```python
from build123d import *

# Parameters (mm, degrees)
BLANKSKE_W              = 85
BLANKSKE_H              = 12.5
BLANK_DEPTH             = 5
TOOTHCUTSIM_DEPTH       = 87.05957239
TEETHCUTS_COUNT         = 12
TEETHCUTS_PITCH         = 7.853981625
ESQUISSE1_R             = 1.025
ENL_V_MAT_EXTRU_1_DEPTH = 87.05957239
ESQUISSE3_W             = 5
ESQUISSE3_H             = 7.71767729
ESQUISSE3_R             = 1.025
BOSS_EXTRU_1_DEPTH      = 7
ESQUISSE4_W             = 7
ESQUISSE4_H             = 7.71767729
BOSS_EXTRU_2_DEPTH      = 10
ESQUISSE5_R             = 1.5
ENL_V_MAT_EXTRU_2_DEPTH = 87.49421946
CONG_1_RADIUS           = 3.858838645
CONG_1_LENGTH           = 7
CONG_2_R                = 1
CONG_3_R                = 1


with BuildPart() as part:
    # BlankSke → Blank (new body)
    with BuildSketch(Plane.XY):
        with Locations((42.5, 6.25)):
            Rectangle(BLANKSKE_W, BLANKSKE_H)
    extrude(amount=-BLANK_DEPTH)

    # TooCutSkeSim → ToothCutSim (cut, through all)
    with BuildSketch(Plane.XY):
        Polygon((1.087088424, 6.875), (-1.087088424, 6.875), (-3.143665836, 12.5254), (3.143665836, 12.5254), align=None)
    toothcutsim = extrude(amount=-TOOTHCUTSIM_DEPTH, mode=Mode.SUBTRACT)

    # TeethCuts: ToothCutSim ×12
    with Locations(*[(i * TEETHCUTS_PITCH, 0, 0) for i in range(1, TEETHCUTS_COUNT)]):
        add(toothcutsim, mode=Mode.SUBTRACT)

    # Esquisse1 → Enlèv. mat.-Extru.1 (cut, through all)
    with BuildSketch(Plane.ZY):
        with Locations((-2.5, 3.4375)):
            Circle(ESQUISSE1_R)
    extrude(amount=-ENL_V_MAT_EXTRU_1_DEPTH, mode=Mode.SUBTRACT)

    # Esquisse3 → Boss.-Extru.1 (add)
    with BuildSketch(Plane(origin=(85, 0, 0), x_dir=(0, 0, -1), z_dir=(1, 0, 0))):
        with Locations((2.5, 3.858838645)):
            Rectangle(ESQUISSE3_W, ESQUISSE3_H)
        with Locations(Location((2.5, 3.4375, 0), (0, 0, 180))):
            Circle(ESQUISSE3_R, mode=Mode.SUBTRACT)
    extrude(amount=BOSS_EXTRU_1_DEPTH)

    # Esquisse4 → Boss.-Extru.2 (add)
    with BuildSketch(Plane.XY):
        with Locations((88.5, 3.858838645)):
            Rectangle(ESQUISSE4_W, ESQUISSE4_H)
    extrude(amount=BOSS_EXTRU_2_DEPTH)

    # Esquisse5 → Enlèv. mat.-Extru.2 (cut, through all)
    with BuildSketch(Plane.ZY.offset(-85)):
        with Locations((5, 3.858838645)):
            Circle(ESQUISSE5_R)
    extrude(amount=-ENL_V_MAT_EXTRU_2_DEPTH, mode=Mode.SUBTRACT)

    # Congé1: full round fillet: the end face becomes a half cylinder, R = half its width
    cong_1_face = Plane((88.5, 3.858838645, 10), x_dir=(-1, 0, 0), z_dir=(0, 0, 1))  # on the end face: x along it, z out of the body
    cong_1_slab = cong_1_face.offset(-CONG_1_RADIUS / 2) * Box(CONG_1_LENGTH, 2 * CONG_1_RADIUS, CONG_1_RADIUS, mode=Mode.PRIVATE)  # the body's end, R deep
    cong_1_round = Plane((88.5, 3.858838645, 6.141161355), x_dir=(0, 0, 1), z_dir=(-1, 0, 0)) * Cylinder(CONG_1_RADIUS, CONG_1_LENGTH, mode=Mode.PRIVATE)  # its axis R under the face
    add(cong_1_slab - cong_1_round, mode=Mode.SUBTRACT)

    # Congé2
    cong_2_edges = [part.edges().sort_by_distance(p)[0] for p in [
        (85, 3.858838645, 0),
    ]]
    fillet(cong_2_edges, radius=CONG_2_R)

    # Congé3
    cong_3_edges = [part.edges().sort_by_distance(p)[0] for p in [
        (92, 3.858838645, -5),
    ]]
    fillet(cong_3_edges, radius=CONG_3_R)


solid = part.part
```
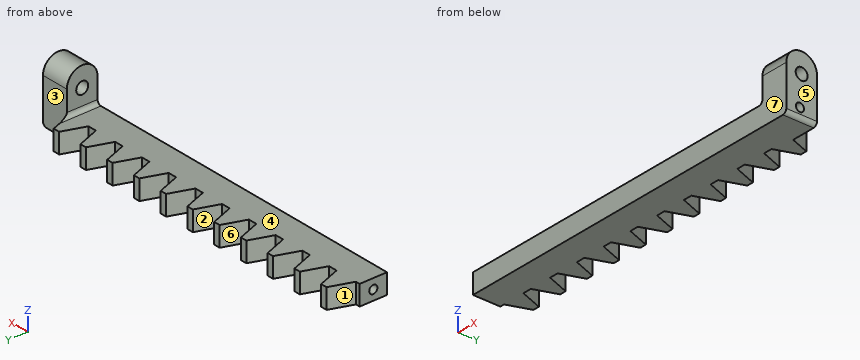
Geometry check sheet. Reference: the model listing, model coordinates, mm. Face numbers are marked on the shaded views. A direction names the side the tool comes from. Round coordinates to 2 decimals unless told otherwise and drop trailing zeros. Loops run counter-clockwise (first coordinate to the right, second up) from the corner with the lowest first, then second, coordinate; pieces in that order, holes last. Notation, with made-up numbers: (71, 34) -> (97, 34) arc R15 cw to (97, 63) -> close; hole circle Ø1 at (15, 59). An arc over 180 degrees is marked (long way). Use a Markdown table: item, result.
(1) Sectioned sample at A-A (z = 5). Enter the section's corners in (x, y).
Calculated:
| item | result |
|---|---|
| outline | (85, 0) -> (92, 0) -> (92, 2.36) -> (85, 2.36) -> close; (85, 5.36) -> (92, 5.36) -> (92, 7.72) -> (85, 7.72) -> close |
(2) Sectioned sample at D-D (z = 8.5). Enter the section's corners in (x, y).
Calculated:
| item | result |
|---|---|
| outline | (85, 0.8) -> (92, 0.8) -> (92, 6.91) -> (85, 6.91) -> close |
(3) Mould release check, pull along X, two halves, no side actions. Record for the marked faces 5, 6 and 7: released by +X, released by -X, zero draft, split by the parting line, or undercut.
Calculated:
| item | result |
|---|---|
| face 5 | released by +X |
| face 6 | undercut |
| face 7 | zero draft |
(4) Go/stop test with flat-tipped pins: P1, Ø2.5, axis at y = 5.5, z = 5, coming from the -X side; P2, Ø1.1, axis at x = 71, z = -2, coming from the +Y side (3 decimals); P3, Ø5.5, axis at x = 90, z = 2, coming from the +Y side. Record where each tip stops, or that it passes through.
Calculated:
| item | result |
|---|---|
| P1 | x = 85 |
| P2 | y = 6.875 |
| P3 | y = 7.72 |
(5) Sectioned sample at C-C (y = 9.25). Give the number of separate pieces and of enclosed holes in the cut face, then the cut area to 3 significant figures.
Calculated:
| item | result |
|---|---|
| separate pieces | 11 |
| enclosed holes | 0 |
| area | 217 mm² |
(6) Set-up check for the marked faces 1, 2, 3 and 4: record each of +Z, -Z, +X, -X, +Y, -Y from which the full face is reachable in a straight line by a thin tool's end or side.
Calculated:
| item | result |
|---|---|
| face 1 | +Z, -Z, -X, +Y |
| face 2 | +Z, -Z, +Y |
| face 3 | +Z, -Z, +X, +Y |
| face 4 | +Z, -X, +Y, -Y |
(7) Scan lines: probe 1 along Y at (x, z) = (47.5, -2.5) (1 decimal); probe 2 along Y at (x, z) = (51, -2.5); probe 3 along Z at (x, y) = (51.5, 4.75). Record each from-to range of solid material in increasing order.
Calculated:
| item | result |
|---|---|
| probe 1 | 0 to 2.4, 4.5 to 6.9 |
| probe 2 | 0 to 2.41, 4.46 to 12.5 |
| probe 3 | -5 to 0 |
